from build123d import *

# Parameters (mm, degrees)
SKETCH1_W            = 49.5
SKETCH1_H            = 49.8
BOSS_EXTRUDE1_DEPTH  = 1.7
M3_CLEARANCE_HOLE1_D = 3.2
LPATTERN1_COUNT      = 2
LPATTERN1_PITCH      = 40
LPATTERN1_COPY_1_D   = 3.2
M3_CLEARANCE_HOLE2_D = 3.2
CHAMFER1_SIZE        = 4


with BuildPart() as part:
    # Sketch1 → Boss-Extrude1 (new body)
    with BuildSketch(Plane(origin=(0, 0, 0), x_dir=(1, 0, 0), z_dir=(0, 1, 0))):
        Rectangle(SKETCH1_W, SKETCH1_H)
    extrude(amount=BOSS_EXTRUDE1_DEPTH)

    # M3 Clearance Hole1 (through all)
    with Locations(Plane(origin=(0, 1.7, 0), x_dir=(1, 0, 0), z_dir=(0, 1, 0))):
        with Locations((-20, 18.7)):
            m3_clearance_hole1 = Hole(M3_CLEARANCE_HOLE1_D / 2)

    # Mirror1: M3 Clearance Hole1 across plane
    add(m3_clearance_hole1.mirror(Plane(origin=(0, 0, 0), x_dir=(0, 0, 1), z_dir=(1, 0, 0))), mode=Mode.SUBTRACT)

    # LPattern1: M3 Clearance Hole1 ×2
    with Locations(*[(0, 0, i * LPATTERN1_PITCH) for i in range(1, LPATTERN1_COUNT)]):
        add(m3_clearance_hole1, mode=Mode.SUBTRACT)

    # LPattern1 copy 1 (through all)
    with Locations(Plane(origin=(0, 1.7, 40), x_dir=(-1, 0, 0), z_dir=(0, 1, 0))):
        with Locations((-20, -18.7)):
            Hole(LPATTERN1_COPY_1_D / 2)

    # M3 Clearance Hole2 (through all)
    with Locations(Plane(origin=(0, 1.7, 0), x_dir=(1, 0, 0), z_dir=(0, 1, 0))):
        with Locations((13.5, -2.4)):
            m3_clearance_hole2 = Hole(M3_CLEARANCE_HOLE2_D / 2)

    # Mirror3: M3 Clearance Hole2 across plane
    add(m3_clearance_hole2.mirror(Plane(origin=(0, 0, 0), x_dir=(0, 0, 1), z_dir=(1, 0, 0))), mode=Mode.SUBTRACT)

    # Chamfer1
    chamfer1_edges = [part.edges().sort_by_distance(p)[0] for p in [
        (24.75, 0.85, 24.9),
        (-24.75, 0.85, 24.9),
        (-24.75, 0.85, -24.9),
        (24.75, 0.85, -24.9),
    ]]
    chamfer(chamfer1_edges, length=CHAMFER1_SIZE)


solid = part.part
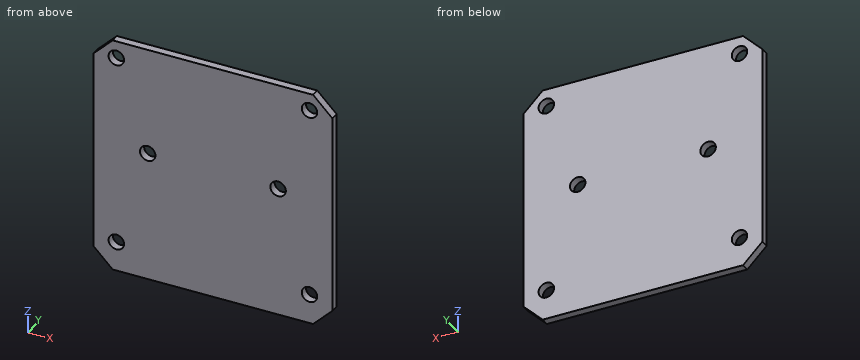
Check sheet for the modelled part. Datum: model origin and axes. Units: mm. Round coordinates to 2 decimals unless told otherwise and drop trailing zeros. Loops run counter-clockwise (first coordinate to the right, second up) from the corner with the lowest first, then second, coordinate; pieces in that order, holes last. Notation, with made-up numbers: M 16.25,-11.5 L 41.25,-11.5 A14 cw 41.25,13.5 Z; hole C 58,68.5 d1. An arc over 180 degrees is marked long. One line per question, with ' | ' between items. Start each with the question number.
Item 1: Section check C-C (y = 1.4). Record the boundary of the cut face in (x, z).
Item 2: Section check B-B (z = 2.4). Record the boundary of the cut face in (x, y).
Item 3: Section check A-A (x = 20). Record the boundary of the cut face in (y, z), and give its area (3 significant figures).
Item 4: Scan lines: probe 1 along Z at (x, y) = (-20, 1.05); probe 2 along Z at (x, y) = (13.5, 0.85); probe 3 along Z at (x, y) = (-19, 0.45). Record each from-to range of solid material in increasing order.
Item 5: Gauge pin test, flat end, axial feed: pin 1 Ø3 at (x, z) = (-20, 21.3) entering from +Y. Record the tip position at first contact, or that the pin passes through.
Item 6: Section check D-D (x = -13.5). Record the boundary of the cut face in (y, z).
Worked out:
1) outline: M -24.75,-20.9 L -20.75,-24.9 L 20.75,-24.9 L 24.75,-20.9 L 24.75,20.9 L 20.75,24.9 L -20.75,24.9 L -24.75,20.9 Z; hole C -20,-18.7 d3.2; hole C -20,21.3 d3.2; hole C -13.5,2.4 d3.2; hole C 13.5,2.4 d3.2; hole C 20,-18.7 d3.2; hole C 20,21.3 d3.2
2) outline: M -24.75,0 L -15.1,0 L -15.1,1.7 L -24.75,1.7 Z; M -11.9,0 L 11.9,0 L 11.9,1.7 L -11.9,1.7 Z; M 15.1,0 L 24.75,0 L 24.75,1.7 L 15.1,1.7 Z
3) outline: M 0,-24.9 L 1.7,-24.9 L 1.7,-20.3 L 0,-20.3 Z; M 0,-17.1 L 1.7,-17.1 L 1.7,19.7 L 0,19.7 Z; M 0,22.9 L 1.7,22.9 L 1.7,24.9 L 0,24.9 Z | area: 73.8 mm^2
4) probe 1: -24.9 to -20.3, -17.1 to 19.7, 22.9 to 24.9 | probe 2: -24.9 to 0.8, 4 to 24.9 | probe 3: -24.9 to -19.95, -17.45 to 20.05, 22.55 to 24.9
5) pin 1: through
6) outline: M 0,-24.9 L 1.7,-24.9 L 1.7,0.8 L 0,0.8 Z; M 0,4 L 1.7,4 L 1.7,24.9 L 0,24.9 Z
